Build history of the part. All positions in model axes, mm. Give positions to 0.01 mm unless a question says otherwise; leave off trailing zeros. Order: outer loops, then holes, each group sorted by start corner. A loop starts at its lowest first (then second) coordinate and runs counter-clockwise, first axis right, second up. Notation, with made-up numbers: (69, 78.5) -> (83, 78.5) arc R20 cw to (83, 113.5) -> close; hole circle Ø7 at (59, -20.75). An arc over 180 degrees is marked (long way). Write item = value, one per line. Start each with the question number.
from build123d import *

# Parameters (mm, degrees)
SKETCH1_W             = 12.5
SKETCH1_H             = 12.5
BOSS_EXTRUDE1_DEPTH   = 60
F_4_0MM_DOWEL_HOLE1_D = 4.5
F_1_0MM_DOWEL_HOLE1_D = 4.5


with BuildPart() as part:
    # Sketch1 → Boss-Extrude1 (new body, symmetric)
    with BuildSketch(Plane(origin=(0, 0, 0), x_dir=(0, 0, -1), z_dir=(1, 0, 0))):
        Rectangle(SKETCH1_W, SKETCH1_H)
    extrude(amount=BOSS_EXTRUDE1_DEPTH, both=True)

    # Ø4.0mm Dowel Hole1 (through all)
    with Locations(Plane.XY.offset(6.25)):
        with Locations((-55, 2.07), (-23, 2.07), (23, 2.07), (55, 2.07)):
            Hole(F_4_0MM_DOWEL_HOLE1_D / 2)

    # Ø1.0mm Dowel Hole1 (through all)
    with Locations(Plane(origin=(0, 6.25, 0), x_dir=(1, 0, 0), z_dir=(0, 1, 0))):
        with Locations((-39, 0), (39, 0), (-7.5, 0), (7.5, 0)):
            Hole(F_1_0MM_DOWEL_HOLE1_D / 2)


solid = part.part
(1) Mould opens along X. For faces 1 (the face through (-5.252, -0.088, -0.099)), 2 (the face through (-60, 0, 0)), 3 (the face through (1, 6.25, 0)), 4 (the face through (60, 0, 0)) say: released by +X, released by -X, zero draft, split by the parting line, or undercut.
(2) Cut at A-A, the plane z = 0. Give the number of separate pieces and of enclosed holes in the cut face, plus the area to 3 significant figures.
(3) Flat gauge pins, fed straight in: P1, Ø6, axis at x = 55, y = 2.07, coming from the -Z side; P2, Ø4, axis at x = -55, y = 2.07, coming from the -Z side. Where does each tip first touch, or does it go through?
(4) Cut at C-C, the plane x = -7.5. Give the cut face in (y, z), plus the area to 3 significant figures.
(5) Wall check: line 1 (X direction, y = -2.5, z = -0.25); line 2 (X direction, y = 3, z = -3.75); line 3 (Y direction, x = -23, z = 3.25). Give the ranges that are in metal, low to high. Write a range as [from, to].
(6) Cut at D-D, the plane y = -4.25. Give the cut face in (x, z), plus the area to 3 significant figures.
Results:
q1.face_1 = undercut
q1.face_2 = released by -X
q1.face_3 = zero draft
q1.face_4 = released by +X
q2.separate_pieces = 5
q2.enclosed_holes = 4
q2.area = 1,210 mm2
q3.P1 = -6.25
q3.P2 = through
q4.outline = (-6.25, -6.25) -> (6.25, -6.25) -> (6.25, -2.25) -> (-6.25, -2.25) -> close; (-6.25, 2.25) -> (6.25, 2.25) -> (6.25, 6.25) -> (-6.25, 6.25) -> close
q4.area = 100 mm2
q5.line_1 = [-60, -41.24], [-36.76, -9.74], [-5.26, 5.26], [9.74, 36.76], [41.24, 60]
q5.line_2 = [-60, -57.05], [-52.95, -25.05], [-20.95, 20.95], [25.05, 52.95], [57.05, 60]
q5.line_3 = [-6.25, -0.18], [4.32, 6.25]
q6.outline = (-60, -6.25) -> (60, -6.25) -> (60, 6.25) -> (-60, 6.25) -> close; hole circle Ø4.5 at (-39, 0); hole circle Ø4.5 at (-7.5, 0); hole circle Ø4.5 at (7.5, 0); hole circle Ø4.5 at (39, 0)
q6.area = 1,440 mm2
